Part model, mm, in its own coordinate system. A direction names the side the tool comes from. Coordinates: 2 decimals unless noted, no trailing zeros. Loops run counter-clockwise (first coordinate to the right, second up) from the corner with the lowest first, then second, coordinate; pieces in that order, holes last. Notation, with made-up numbers: (33.5, 82.25) -> (83.5, 82.25) arc R24 ccw to (83.5, 119.25) -> close; hole circle Ø8 at (-14.5, 33.25). An arc over 180 degrees is marked (long way). Use one line per item in the form item = value. Start each with the question number.
(1) Band-saw the part on A-A on z = -14. Give the cut face in (x, y), then the cut area to 3 significant figures.
(2) Band-saw the part on B-B on z = -32. Give the cut face in (x, y).
(3) 3-axis set-ups, long thin cutter, end or side, ignore diameter. For faces 1 (the flat face through (-8.874, -15.661, -14.956)), 2 (the flat face through (-10, 10, -36)), 3 (the flat face through (-9.126, 15.516, -14.956)), 4 (the flat face through (12, 15, -30)), 5 (the flat face through (-18, 0, -15)): which of +Z, -Z, +X, -X, +Y, -Y reach the whole face in a straight line?
(4) Pin check, flat tips, straight feed: P1, Ø6, axis at y = 1.5, z = -12.5, coming from the -X side; P2, Ø1.5, axis at x = -1, z = -11.5, coming from the -Y side; P3, Ø21.5, axis at x = 0, y = 0, coming from the -Z side. Stop position of each tip, or through.
(5) Mould opens along Y. For faces 6 (the flat face through (18, 0, -15)), 7 (the cylindrical face through (10, 3.2, -18.2)), 8 (the conical face through (-16.197, 9.299, -0.583)) say: +Y half, -Y half, draft (parallel to the pull), parting line (faces both ways), or undercut.
(6) Drill centre lines: L1, parallel to X at y = 1.5, z = -6.5; L2, parallel to X at y = -6, z = -15; L3, parallel to Z at x = -7, y = 20. Where is each one in solid material? Low to high. Write a range as [from, to].
```python
from build123d import *

# Parameters (mm, degrees)
BASENUT_START = -36
BASENUTSKE_R  = 10.5
BASENUT_DEPTH = 36
COLLARSKE_W   = 6
COLLARSKE_H   = 12
FILLET_2_R    = 0.5


# Read off the part's stored shape, not the designer's step: ThreadSchematic
with BuildPart() as part:
    # BaseNutSke → BaseNut (new body)
    with BuildSketch(Plane.XY.offset(BASENUT_START)):
        Polygon((18, 10.392304845), (18, -10.392304845), (0, -20.784609691), (-18, -10.392304845), (-18, 10.392304845), (0, 20.784609691), align=None)
        Circle(BASENUTSKE_R, mode=Mode.SUBTRACT)
    extrude(amount=BASENUT_DEPTH)

    # Sketch5 (on Right Plane) → EndChamfer (revolve, cut)
    with BuildSketch(Plane(origin=(0, 0, 0), x_dir=(0, 0, -1), z_dir=(1, 0, 0))):
        Polygon((35.9746, 12), (34.819257562, 10.35), (36.0254, 10.35), (36.0254, 12), align=None)
    revolve(axis=Axis((0, 10.35, -36.0254), (0, 0, 1)), mode=Mode.SUBTRACT)

    # CollarSke → Collar (revolve)
    with BuildSketch(Plane(origin=(0, 0, 0), x_dir=(0, 0, -1), z_dir=(1, 0, 0)), mode=Mode.PRIVATE) as collar_sk:
        with Locations((33, 16.5)):
            Rectangle(COLLARSKE_W, COLLARSKE_H)
    revolve(collar_sk.sketch.rotate(Axis((0, 0, 0), (0, 0, -1)), 90), axis=Axis((0, 0, 0), (0, 0, -1)))

    # Sketch3 → Chamfer 2 (revolve, cut)
    with BuildSketch(Plane(origin=(0, 0, 0), x_dir=(0, 0, -1), z_dir=(1, 0, 0))):
        Polygon((2.4, 33.484609691), (-12.7, 33.484609691), (-12.7, 18), (0, 18), (2.4, 20.784609691), align=None)
    revolve(axis=Axis((0, 0, 0), (0, 0, -1)), mode=Mode.SUBTRACT)

    # ThreadSchematic outline → ThreadSchematic (revolve, cut)
    with BuildSketch(Plane.XZ):
        Polygon((10.5, 0), (10.5, -1.050311307), (12, 0), align=None)
        Polygon((12, -35.9746), (10.5, -34.924288693), (10.5, -36), (12, -36), align=None)
    revolve(axis=Axis((0, 0, 0), (0, 0, 1)), mode=Mode.SUBTRACT)

    # Fillet 2
    fillet_2_edges = [part.edges().sort_by_distance(p)[0] for p in [
        (9, 15.588457268, -30),
        (-9, 15.588457268, -30),
        (-18, 0, -30),
        (-9, -15.588457268, -30),
        (9, -15.588457268, -30),
        (18, 0, -30),
    ]]
    fillet(fillet_2_edges, radius=FILLET_2_R)


solid = part.part
```
A:
q1.outline = (-18, -10.39) -> (0, -20.78) -> (18, -10.39) -> (18, 10.39) -> (0, 20.78) -> (-18, 10.39) -> close; hole circle Ø21 at (0, 0)
q1.area = 776 mm²
q2.outline = circle Ø45 at (0, 0); hole circle Ø21 at (0, 0)
q3.face_1 = +Z, -X, -Y
q3.face_2 = -Z, +X, -X, +Y, -Y
q3.face_3 = +Z, -X, +Y
q3.face_4 = +Z
q3.face_5 = +Z, -X, +Y, -Y
q4.P1 = -18
q4.P2 = -20.64
q4.P3 = -35.1
q5.face_6 = draft
q5.face_7 = undercut
q5.face_8 = +Y half
q6.L1 = [-18, -10.39], [10.39, 18]
q6.L2 = [-18, -8.62], [8.62, 18]
q6.L3 = [-36, -30]
